from build123d import *

# Parameters (mm, degrees)
SKETCH1_R           = 9
BOSS_EXTRUDE1_DEPTH = 20
SKETCH2_R           = 3
CUT_EXTRUDE1_DEPTH  = 52
SKETCH3_R           = 14
BOSS_EXTRUDE2_DEPTH = 8
SKETCH4_R           = 3
CUT_EXTRUDE2_DEPTH  = 12


with BuildPart() as part:
    # Sketch1 → Boss-Extrude1 (new body)
    with BuildSketch(Plane(origin=(0, 0, 0), x_dir=(1, 0, 0), z_dir=(0, 1, 0))):
        Circle(SKETCH1_R)
    extrude(amount=BOSS_EXTRUDE1_DEPTH)

    # Sketch2 → Cut-Extrude1 (cut)
    with BuildSketch(Plane.XZ):
        Circle(SKETCH2_R)
    extrude(amount=-CUT_EXTRUDE1_DEPTH, mode=Mode.SUBTRACT)

    # Sketch3 → Boss-Extrude2 (add)
    with BuildSketch(Plane(origin=(0, 20, 0), x_dir=(1, 0, 0), z_dir=(0, 1, 0))):
        Circle(SKETCH3_R)
    extrude(amount=BOSS_EXTRUDE2_DEPTH)

    # Sketch4 → Cut-Extrude2 (cut)
    with BuildSketch(Plane(origin=(0, 28, 0), x_dir=(1, 0, 0), z_dir=(0, 1, 0))):
        Circle(SKETCH4_R)
    extrude(amount=-CUT_EXTRUDE2_DEPTH, mode=Mode.SUBTRACT)


solid = part.part
For this review, take the finished solid that the model builds, in its own axes (mm). A direction names the side the tool comes from. Coordinates: 2 decimals unless noted, no trailing zeros. Loops run counter-clockwise (first coordinate to the right, second up) from the corner with the lowest first, then second, coordinate; pieces in that order, holes last. Notation, with made-up numbers: (53.5, 66.5) - (92.5, 66.5) arc R26 ccw to (92.5, 98.5) - close; hole circle Ø2 at (1, -10.5). An arc over 180 degrees is marked (long way). Use a Markdown table: item, result. Add a question column.
Item 1: Mouldability with a two-part tool opening along Z and no side actions: class faces 1 (the face through (12.932, 23.944, 5.362)), 2 (the face through (0, 0, 4)), 3 (the face through (-3, 14, 0)) as pulls with the +Z half, pulls with the -Z half, needs draft (parallel to the pull), parting line crosses it, or undercut.
Item 2: We need section C-C (y = 8.25). Give the boundary of the cut face in (x, z), and give its area (3 significant figures).
Item 3: We need section A-A (x = 0). Give the boundary of the cut face in (y, z).
Item 4: Tool access review of faces 4 (the face through (-0.2, 28, -3.3)), 5 (the face through (-1.172, 9.86, -8.923)): name each direction out of +Z, -Z, +X, -X, +Y, -Y from which nothing blocks a thin tool from reaching the whole face with its end or side.
Item 5: We need section B-B (z = 0). Give the boundary of the cut face in (x, y), and give its area (3 significant figures).
Item 6: Insertion check: pin 1 Ø5.5 at (x, z) = (0, 0) entering from +Y; pin 2 Ø12 at (x, y) = (9.5, 20.5) entering from +Z; pin 3 Ø6 at (x, y) = (5, 10.5) entering from +Z; pin 4 Ø12 at (y, z) = (8.5, 6.5) entering from -X. Each pin has a flat end and moves straight along its axis. Give the tip position at first contact, or say it passes through.
Item 7: We need section D-D (x = -6). Give the boundary of the cut face in (y, z), and give its area (3 significant figures).
Item 8: For line 1 (X direction, y = 14.75, z = 0); line 2 (Z direction, x = 0, y = 20.25), list the stretches that pass through material, from the lowest coordinate up.
Results list:
| question | item | result |
|---|---|---|
| 1 | face 1 | parting line crosses it |
| 1 | face 2 | needs draft |
| 1 | face 3 | undercut |
| 2 | outline | circle Ø18 at (0, 0); hole circle Ø6 at (0, 0) |
| 2 | area | 226 mm^2 |
| 3 | outline | (0, -9) - (20, -9) - (20, -14) - (28, -14) - (28, -3) - (0, -3) - close; (0, 3) - (28, 3) - (28, 14) - (20, 14) - (20, 9) - (0, 9) - close |
| 4 | face 4 | +Z, -Z, +X, -X, +Y |
| 4 | face 5 | -Y |
| 5 | outline | (-14, 20) - (-9, 20) - (-9, 0) - (-3, 0) - (-3, 28) - (-14, 28) - close; (3, 0) - (9, 0) - (9, 20) - (14, 20) - (14, 28) - (3, 28) - close |
| 5 | area | 416 mm^2 |
| 6 | pin 1 | passes through |
| 6 | pin 2 | stops at z = 13.56 |
| 6 | pin 3 | stops at z = 8.77 |
| 6 | pin 4 | stops at x = -8.99 |
| 7 | outline | (0, -6.71) - (20, -6.71) - (20, -12.65) - (28, -12.65) - (28, 12.65) - (20, 12.65) - (20, 6.71) - (0, 6.71) - close |
| 7 | area | 471 mm^2 |
| 8 | line 1 | x = -9 to -3, 3 to 9 |
| 8 | line 2 | z = -14 to -3, 3 to 14 |
